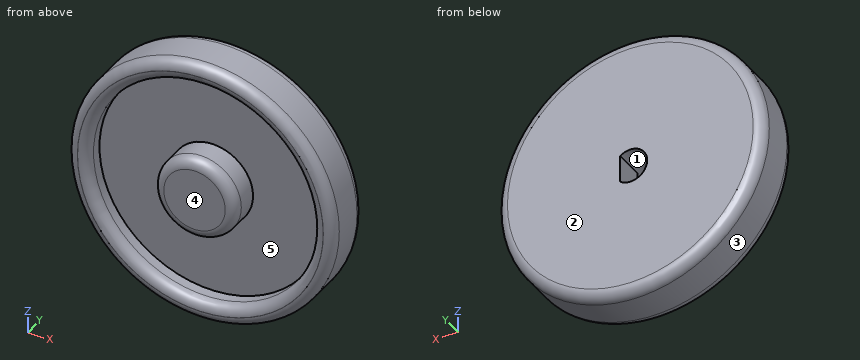
from build123d import *

# Parameters (mm, degrees)
CYLINDER236_R     = 11
CYLINDER236_DEPTH = 2
CYLINDER235_R     = 1.65
CYLINDER235_DEPTH = 5
CYLINDER234_R     = 13
CYLINDER234_DEPTH = 5
BOX161_W          = 10
BOX161_H          = 12
BOX161_DEPTH      = 10
CYLINDER233_R     = 1.65
CYLINDER233_DEPTH = 5
FILLET067_R       = 0.99
FILLET066_R       = 1
CYLINDER232_R     = 1.65
CYLINDER232_DEPTH = 2
CYLINDER231_R     = 4
CYLINDER231_DEPTH = 3
FILLET065_R       = 1


with BuildPart() as cylinder519:
    # Cylinder236 → Cylinder236 (new body)
    with BuildSketch(Plane(origin=(333.25, -23, -34.25), x_dir=(1, 0, 0), z_dir=(0, -1, 0))):
        Circle(CYLINDER236_R)
    extrude(amount=CYLINDER236_DEPTH)


with BuildPart() as cylinder517:
    # Cylinder235 → Cylinder235 (new body)
    with BuildSketch(Plane(origin=(333.25, -20, -34.25), x_dir=(1, 0, 0), z_dir=(0, -1, 0))):
        Circle(CYLINDER235_R)
    extrude(amount=CYLINDER235_DEPTH)


with BuildPart() as cut172:
    # Cylinder234 → Cylinder234 (new body)
    with BuildSketch(Plane(origin=(333.25, -20, -34.25), x_dir=(1, 0, 0), z_dir=(0, -1, 0))):
        Circle(CYLINDER234_R)
    extrude(amount=CYLINDER234_DEPTH)

    # Cut172: cut Cylinder517
    add(cylinder517.part, mode=Mode.SUBTRACT)


with BuildPart() as cube257:
    # Box161 → Box161 (new body)
    with BuildSketch(Plane(origin=(320.25, -4, -55), x_dir=(1, 0, 0), z_dir=(0, 0, 1))):
        with Locations((5, 6)):
            Rectangle(BOX161_W, BOX161_H)
    extrude(amount=BOX161_DEPTH)


with BuildPart() as fillet066:
    # Cylinder233 → Cylinder233 (new body)
    with BuildSketch(Plane(origin=(329.25, 8, -49), x_dir=(1, 0, 0), z_dir=(0, -1, 0))):
        Circle(CYLINDER233_R)
    extrude(amount=CYLINDER233_DEPTH)

    # Cut171: cut Cube257
    add(cube257.part, mode=Mode.SUBTRACT)


with BuildPart() as fillet066_1:
    # Cut171 placement: moved
    add(fillet066.part.moved(Location((4, -28, 14.75))))

    # Fusion199: union Cut172
    add(cut172.part)

    # Cut170: cut Cylinder519
    add(cylinder519.part, mode=Mode.SUBTRACT)

    # Fillet067
    fillet067_edges = [fillet066_1.edges().sort_by_distance(p)[0] for p in [
        (320.25, -25, -34.25),
        (322.25, -25, -34.25),
    ]]
    fillet(fillet067_edges, radius=FILLET067_R)

    # Fillet066
    fillet066_edges = [fillet066_1.edges().sort_by_distance(p)[0] for p in [
        (320.25, -20, -34.25),
    ]]
    fillet(fillet066_edges, radius=FILLET066_R)


with BuildPart() as cylinder520:
    # Cylinder232 → Cylinder232 (new body)
    with BuildSketch(Plane(origin=(333.25, -23, -34.25), x_dir=(1, 0, 0), z_dir=(0, -1, 0))):
        Circle(CYLINDER232_R)
    extrude(amount=CYLINDER232_DEPTH)


with BuildPart() as supports_wheel:
    # Cylinder231 → Cylinder231 (new body)
    with BuildSketch(Plane(origin=(333.25, -23, -34.25), x_dir=(1, 0, 0), z_dir=(0, -1, 0))):
        Circle(CYLINDER231_R)
    extrude(amount=CYLINDER231_DEPTH)

    # Cut169: cut Cylinder520
    add(cylinder520.part, mode=Mode.SUBTRACT)

    # Fillet065
    fillet065_edges = [supports_wheel.edges().sort_by_distance(p)[0] for p in [
        (329.25, -26, -34.25),
    ]]
    fillet(fillet065_edges, radius=FILLET065_R)

    # Fusion198: union Fillet066
    add(fillet066_1.part)


with BuildPart() as supports_wheel_1:
    # Fusion198 placement: moved
    add(supports_wheel.part.moved(Location((-78.7, -9, 17.5))))


solid = supports_wheel_1.part
Check sheet for the modelled part. Datum: model origin and axes. Units: mm. Face numbers are marked on the shaded views. A direction names the side the tool comes from. Coordinates: 2 decimals unless noted, no trailing zeros. Loops run counter-clockwise (first coordinate to the right, second up) from the corner with the lowest first, then second, coordinate; pieces in that order, holes last. Notation, with made-up numbers: (-6.5, 66) -> (10.5, 66) arc R12 ccw to (10.5, 74) -> close; hole circle Ø2 at (14, 17). An arc over 180 degrees is marked (long way). Write item = value, one per line. Start each with the question number.
1. Depth check by flat-ended pin: P1, Ø6, axis at x = 255, z = -22.5, coming from the -Y side; P2, Ø1, axis at x = 256.5, y = -32, coming from the -Z side; P3, Ø1.5, axis at x = 246, z = -24, coming from the -Y side; P4, Ø1.5, axis at x = 260, y = -33.5, coming from the -Z side. Enter the tip coordinate at first touch or a pass-through.
2. Material ranges on line 1 (Z direction, x = 254.55, y = -32.2); line 2 (Y direction, x = 256, z = -24); line 3 (Z direction, x = 254.55, y = -30.5), recorded low to high.
3. Tool access check on the marked faces 4 and 5. Record the directions out of +Z, -Z, +X, -X, +Y, -Y that give a thin tool (end or side, any length) a straight path to the whole face; none if there is none.
4. Section check C-C on y = -29.5. Record the cut outline in (x, z), then the cut area to 3 significant figures.
5. Draft check along Z on the marked faces 1, 2 and 3. Enter one of: released by +Z, released by -Z, zero draft, split by the parting line, or undercut.
Responses:
q1.P1 = -35
q1.P2 = -29.67
q1.P3 = -34
q1.P4 = -28.83
q2.line_1 = -29.75 to -27.75, -20.75 to -18.4, -15.1 to -12.75, -5.75 to -3.75
q2.line_2 = -32 to -29
q2.line_3 = -29.75 to -18.4, -15.1 to -3.75
q3.face_4 = +Z, -Z, +X, -X, -Y
q3.face_5 = -Y
q4.outline = circle Ø25.73 at (254.55, -16.75); hole (255.55, -18.06) -> (255.55, -15.44) arc R1.65 ccw (long way) to start
q4.area = 513 mm2
q5.face_1 = undercut
q5.face_2 = zero draft
q5.face_3 = split by the parting line
